Can you work these out from the drawing? Everything is in mm from the part's minimum corner. A direction names the side the tool comes from. Round coordinates to 2 decimals unless told otherwise and drop trailing zeros. Write each loop counter-clockwise with the first axis right and the second up, starting at its lowest first coordinate (ties: lowest second). Pieces come first, ordered by that corner, then holes. Notation, with made-up numbers: (-9.75, 69) -> (6.25, 69) arc R17 ccw to (6.25, 101) -> close; hole circle Ø7 at (79, -17). An arc over 180 degrees is marked (long way). Put each result on its own line as item: value. Start each with the question number.
1. We'd pull the mould along Z, two halves only. Please class the marked faces 3, 4 and 5: +Z half, -Z half, draft (parallel to the pull), parting line (faces both ways), or undercut.
2. Which directions (+Z, -Z, +X, -X, +Y, -Y) give clear straight access to the entire face, cutting with the end or side of a thin tool? Please do the marked faces 1 and 2.
3. Suppose I cut it at A-A (x = 21.5). Please give me the cut outline in (y, z).
4. For pin 1 (6 mm diameter, centred on y = 8.5, z = 8, fed in from +X); pin 2 (2 mm diameter, centred on x = 21.5, y = 11.5, fed in from +Z); pin 3 (2.5 mm diameter, centred on x = 25, y = 18, fed in from +Z), each with a flat end and sliding along its axis, tell me the tip position at first contact or that it passes through.
5. I need wall thicknesses on probe 1 along Y at (x, z) = (22.5, 1.15); probe 2 along X at (y, z) = (22, 2) (1 decimal); probe 3 along Z at (x, y) = (38, 14). Which ranges of each line are inside material? Lowest first, please. Write a range as from..to.
6. Suppose I cut it at D-D (z = 28). Please give me the cut outline in (x, y).
7. Suppose I cut it at B-B (y = 6.5). Please give me the cut outline in (x, z).
8. Suppose I cut it at C-C (x = 6). Please give me the cut outline in (y, z).
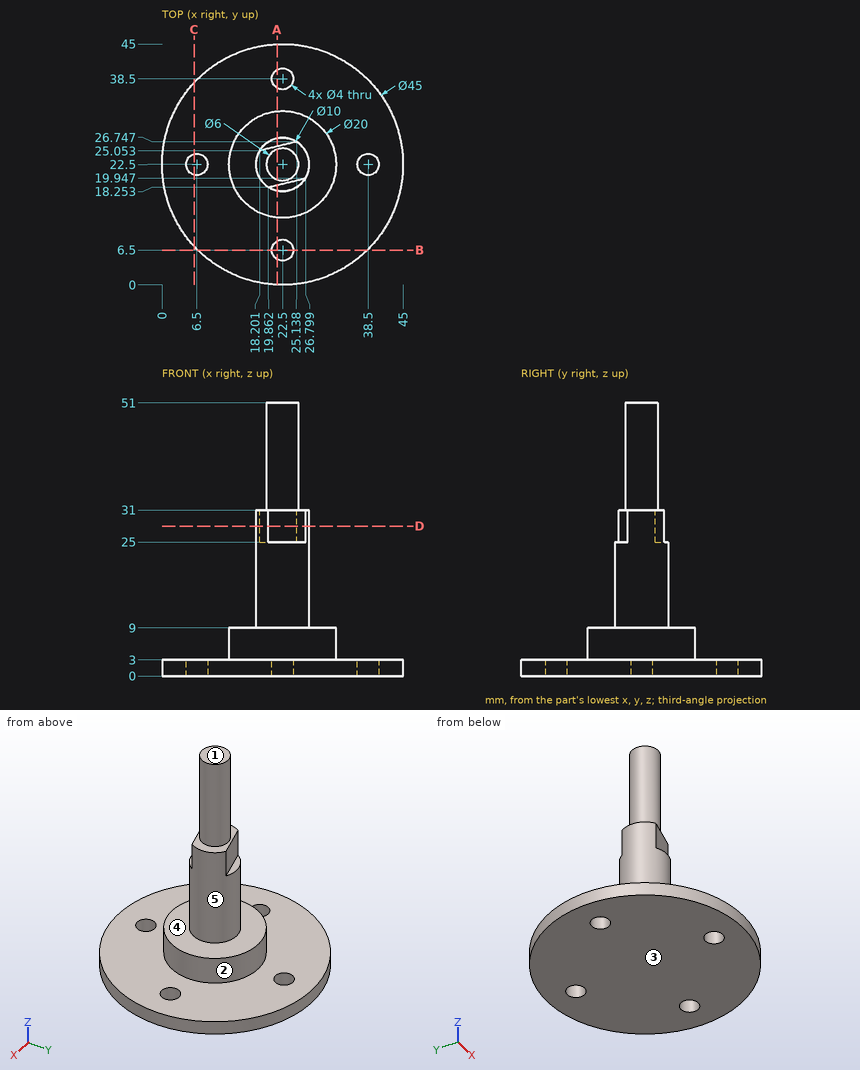
Verdict:
1. face 3: -Z half
1. face 4: +Z half
1. face 5: draft
2. face 1: +Z, +X, -X, +Y, -Y
2. face 2: +Z
3. outline: (0.02, 0) -> (4.77, 0) -> (4.77, 3) -> (0.02, 3) -> close; (8.23, 0) -> (36.77, 0) -> (36.77, 3) -> (32.45, 3) -> (32.45, 9) -> (27.4, 9) -> (27.4, 25) -> (25.86, 25) -> (25.86, 31) -> (25.33, 31) -> (25.33, 51) -> (19.67, 51) -> (19.67, 31) -> (18.65, 31) -> (18.65, 25) -> (17.6, 25) -> (17.6, 9) -> (12.55, 9) -> (12.55, 3) -> (8.23, 3) -> close; (40.23, 0) -> (44.98, 0) -> (44.98, 3) -> (40.23, 3) -> close
4. pin 1: passes through
4. pin 2: stops at z = 3
4. pin 3: stops at z = 25
5. probe 1: y = 0..4.5, 8.5..36.5, 40.5..45
5. probe 2: x = 0..4.6, 8.4..36.6, 40.4..45
5. probe 3: z = 0..3
6. outline: (18.2, 25.05) arc R5 ccw to (19.86, 18.25) -> (26.8, 19.95) arc R5 ccw to (25.14, 26.75) -> close
7. outline: (6.68, 0) -> (20.5, 0) -> (20.5, 3) -> (6.68, 3) -> close; (24.5, 0) -> (38.32, 0) -> (38.32, 3) -> (24.5, 3) -> close
8. outline: (7.2, 0) -> (20.56, 0) -> (20.56, 3) -> (7.2, 3) -> close; (24.44, 0) -> (37.8, 0) -> (37.8, 3) -> (24.44, 3) -> close
